Autodesk Inventor part; units mm, degrees
ref_plane "YZ Plane" through (0, 0, 0) normal (1, 0, 0) x (0, 1, 0)
ref_plane "XZ Plane" through (0, 0, 0) normal (0, 1, 0) x (-1, 0, 0)
ref_plane "XY Plane" through (0, 0, 0) normal (0, 0, 1) x (1, 0, 0)
sketch "Sketch1" plane through (0, 0, 0) normal (0, 0, 1) x (1, 0, 0)
  line L0 (-9.652, -11.176) -> (9.652, -11.176)
  arc A0 (-11.176, -9.652) -> (-9.652, -11.176) centre (-9.652, -9.652) ccw
  line L1 (-11.176, 9.652) -> (-11.176, -9.652)
  arc A1 (-9.652, 11.176) -> (-11.176, 9.652) centre (-9.652, 9.652) ccw
  line L2 (9.652, 11.176) -> (-9.652, 11.176)
  arc A2 (11.176, 9.652) -> (9.652, 11.176) centre (9.652, 9.652) ccw
  line L3 (11.176, -9.652) -> (11.176, 9.652)
  arc A3 (9.652, -11.176) -> (11.176, -9.652) centre (9.652, -9.652) ccw
  arc A4 (-6.731, 12.7) -> (-6.35, 13.081) centre (-6.731, 13.081) ccw
  line L4 (-6.731, 12.7) -> (-10.5918, 12.7)
  arc A5 (-10.5918, 12.7) -> (-12.7, 10.5918) centre (-10.5918, 10.5918) ccw
  line L5 (-12.7, 10.5918) -> (-12.7, 6.731)
  arc A6 (-13.081, 6.35) -> (-12.7, 6.731) centre (-13.081, 6.731) ccw
  line L6 (-13.081, 6.35) -> (-25.019, 6.35)
  arc A7 (-25.019, 6.35) -> (-25.4, 5.969) centre (-25.019, 5.969) ccw
  line L7 (-25.4, 5.969) -> (-25.4, 4.826)
  arc A8 (-25.4, 4.826) -> (-24.638, 4.064) centre (-24.638, 4.826) ccw
  line L8 (-24.638, 4.064) -> (-23.0632, 4.064)
  arc A9 (-23.0632, 4.064) -> (-22.6822, 4.445) centre (-23.0632, 4.445) ccw
  arc A10 (-22.3012, 4.826) -> (-22.6822, 4.445) centre (-22.3012, 4.445) ccw
  line L9 (-22.3012, 4.826) -> (-13.081, 4.826)
  arc A11 (-12.7, 4.445) -> (-13.081, 4.826) centre (-13.081, 4.445) ccw
  line L10 (-12.7, 4.445) -> (-12.7, -4.445)
  arc A12 (-13.081, -4.826) -> (-12.7, -4.445) centre (-13.081, -4.445) ccw
  line L11 (-13.081, -4.826) -> (-22.3012, -4.826)
  arc A13 (-22.6822, -4.445) -> (-22.3012, -4.826) centre (-22.3012, -4.445) ccw
  arc A14 (-22.6822, -4.445) -> (-23.0632, -4.064) centre (-23.0632, -4.445) ccw
  line L12 (-23.0632, -4.064) -> (-24.638, -4.064)
  arc A15 (-24.638, -4.064) -> (-25.4, -4.826) centre (-24.638, -4.826) ccw
  line L13 (-25.4, -4.826) -> (-25.4, -5.969)
  arc A16 (-25.4, -5.969) -> (-25.019, -6.35) centre (-25.019, -5.969) ccw
  line L14 (-25.019, -6.35) -> (-13.081, -6.35)
  arc A17 (-12.7, -6.731) -> (-13.081, -6.35) centre (-13.081, -6.731) ccw
  line L15 (-12.7, -6.731) -> (-12.7, -10.5918)
  arc A18 (-12.7, -10.5918) -> (-10.5918, -12.7) centre (-10.5918, -10.5918) ccw
  line L16 (-10.5918, -12.7) -> (10.5918, -12.7)
  arc A19 (10.5918, -12.7) -> (12.7, -10.5918) centre (10.5918, -10.5918) ccw
  line L17 (12.7, -10.5918) -> (12.7, 10.5918)
  arc A20 (12.7, 10.5918) -> (10.5918, 12.7) centre (10.5918, 10.5918) ccw
  line L18 (10.5918, 12.7) -> (6.731, 12.7)
  arc A21 (6.35, 13.081) -> (6.731, 12.7) centre (6.731, 13.081) ccw
  line L19 (6.35, 13.081) -> (6.35, 25.019)
  arc A22 (6.35, 25.019) -> (5.969, 25.4) centre (5.969, 25.019) ccw
  line L20 (5.969, 25.4) -> (4.826, 25.4)
  arc A23 (4.826, 25.4) -> (4.064, 24.638) centre (4.826, 24.638) ccw
  line L21 (4.064, 24.638) -> (4.064, 23.0632)
  arc A24 (4.064, 23.0632) -> (4.445, 22.6822) centre (4.445, 23.0632) ccw
  arc A25 (4.826, 22.3012) -> (4.445, 22.6822) centre (4.445, 22.3012) ccw
  line L22 (4.826, 22.3012) -> (4.826, 13.081)
  arc A26 (4.445, 12.7) -> (4.826, 13.081) centre (4.445, 13.081) ccw
  line L23 (4.445, 12.7) -> (-4.445, 12.7)
  arc A27 (-4.826, 13.081) -> (-4.445, 12.7) centre (-4.445, 13.081) ccw
  line L24 (-4.826, 13.081) -> (-4.826, 22.3012)
  arc A28 (-4.445, 22.6822) -> (-4.826, 22.3012) centre (-4.445, 22.3012) ccw
  arc A29 (-4.445, 22.6822) -> (-4.064, 23.0632) centre (-4.445, 23.0632) ccw
  line L25 (-4.064, 23.0632) -> (-4.064, 24.638)
  arc A30 (-4.064, 24.638) -> (-4.826, 25.4) centre (-4.826, 24.638) ccw
  line L26 (-4.826, 25.4) -> (-5.969, 25.4)
  arc A31 (-5.969, 25.4) -> (-6.35, 25.019) centre (-5.969, 25.019) ccw
  line L27 (-6.35, 25.019) -> (-6.35, 13.081)
  point P0 (0, 0)
extrude "Extrusion1" add sketch "Sketch1" against normal blind 304.8
properties part number "9030"
Work out the finished part from the listing and answer in its coordinate system (mm). A direction names the side the tool comes from. Coordinates: 2 decimals unless noted, no trailing zeros. Loops run counter-clockwise (first coordinate to the right, second up) from the corner with the lowest first, then second, coordinate; pieces in that order, holes last. Notation, with made-up numbers: (-23.75, -33) -> (10.25, -33) arc R19 ccw to (10.25, -12) -> close; hole circle Ø10 at (15, -38). An arc over 180 degrees is marked (long way). Write each question's results on one line, items separated by ' | '. Start each with the question number.
1) Consider line 1 along Y through (x, z) = (10, -224.5); line 2 along Y through (x, z) = (-14, -59); line 3 along X through (y, z) = (-7, -206). Determine where each line is inside the solid, lowest interval first.
2) Flat-ended cylindrical pins translate along their axes: P1, Ø0.8, axis at x = -23.5, z = -154.5, coming from the -Y side; P2, Ø10, axis at x = -16.5, z = -129, coming from the -Y side; P3, Ø0.8, axis at y = 23.5, z = -123, coming from the -X side. Find the tip coordinate at first contact, or state that the pin passes through.
3) For faces 5 (the flat face through (6.35, 19, -150)), 6 (the flat face through (-18, 4.826, -150)), 7 (the flat face through (-19, -6.35, -150)), determine the directions among +Z, -Z, +X, -X, +Y, -Y from which every point of the face is accessible in a straight line to the end or side of a thin tool.
4) Find section A-A on x = -18. Determine the outline of the cut face in (y, z).
5) The mould has two halves that part along X. Classify faces 1 (the flat face through (-18, -4.826, -150)), 2 (the flat face through (0, -11.176, -150)), 3 (the flat face through (-6.35, 19, -150)), 4 (the flat face through (-4, 12, 0)): pulls with the +X half, pulls with the -X half, needs draft (parallel to the pull), parting line crosses it, or undercut.
Response values:
1) line 1: y = -12.7 to -11.14, 11.14 to 12.7 | line 2: y = -6.35 to -4.83, 4.83 to 6.35 | line 3: x = -12.7 to -11.18, 11.18 to 12.7
2) P1: stops at y = -6.35 | P2: stops at y = -12.49 | P3: stops at x = -6.35
3) face 5: +Z, -Z, +X, +Y | face 6: +Z, -Z | face 7: +Z, -Z, -X, -Y
4) outline: (-6.35, -304.8) -> (-4.83, -304.8) -> (-4.83, 0) -> (-6.35, 0) -> close; (4.83, -304.8) -> (6.35, -304.8) -> (6.35, 0) -> (4.83, 0) -> close
5) face 1: undercut | face 2: undercut | face 3: pulls with the -X half | face 4: needs draft
